Here's the drawing with two shaded views (mm, measured from the low corner). I have some questions. A direction names the side the tool comes from. Round coordinates to 2 decimals unless told otherwise and drop trailing zeros. Loops run counter-clockwise (first coordinate to the right, second up) from the corner with the lowest first, then second, coordinate; pieces in that order, holes last. Notation, with made-up numbers: (46.25, 24.25) -> (78.25, 24.25) arc R36 ccw to (78.25, 61.25) -> close; hole circle Ø3 at (20.5, 83). An arc over 180 degrees is marked (long way). Write item = value, one per line.
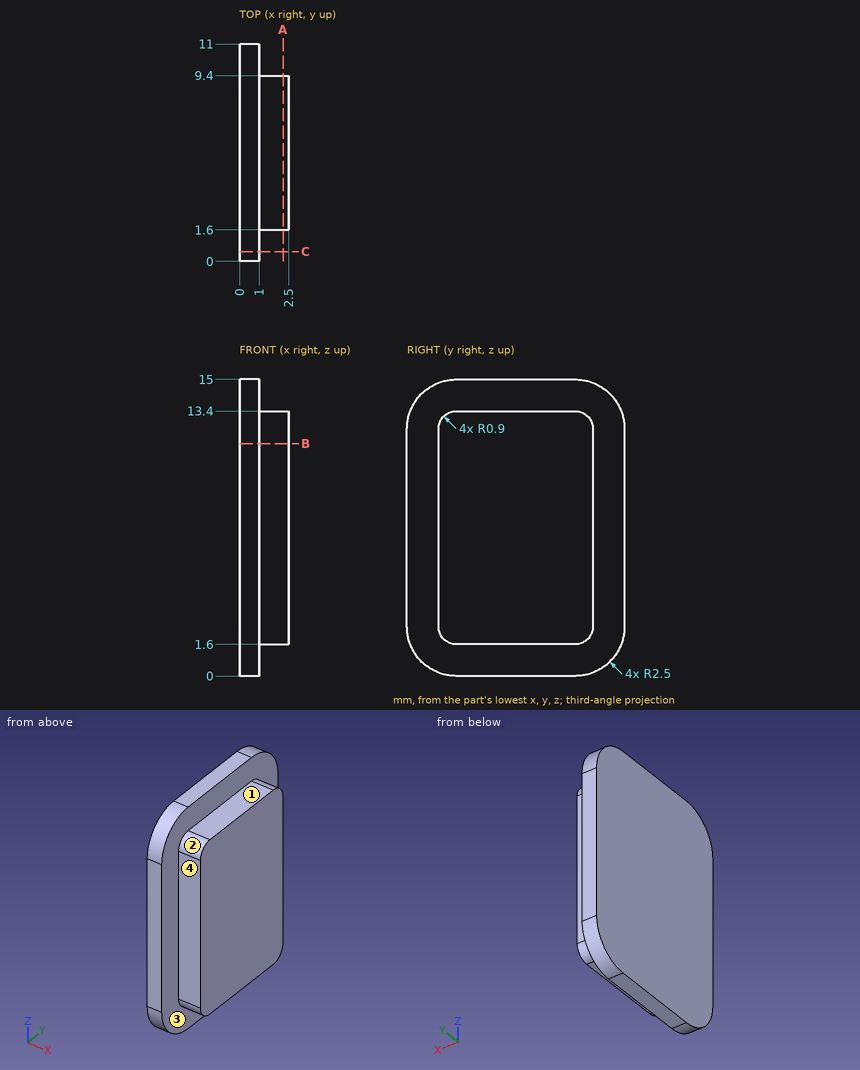
1. Suppose I cut it at C-C, the plane y = 0.5. List the corners of the cut face in (x, z) for me, and give its area (3 significant figures).
Entries:
outline = (0, 1) -> (1, 1) -> (1, 14) -> (0, 14) -> close
area = 13.0 mm²
2. Suppose I cut it at A-A, the plane x = 2.2. List the corners of the cut face in (y, z) for me, and give its area (3 significant figures).
Entries:
outline = (1.6, 2.5) arc R0.9 ccw to (2.5, 1.6) -> (8.5, 1.6) arc R0.9 ccw to (9.4, 2.5) -> (9.4, 12.5) arc R0.9 ccw to (8.5, 13.4) -> (2.5, 13.4) arc R0.9 ccw to (1.6, 12.5) -> close
area = 91.3 mm²
3. Suppose I cut it at B-B, the plane z = 11.75. List the corners of the cut face in (x, y) for me, and give its area (3 significant figures).
Entries:
outline = (0, 0) -> (1, 0) -> (1, 1.6) -> (2.5, 1.6) -> (2.5, 9.4) -> (1, 9.4) -> (1, 11) -> (0, 11) -> close
area = 22.7 mm²
4. I need wall thicknesses on line 1 (Y direction, x = 1.85, z = 6.75); line 2 (X direction, y = 1, z = 3.5); line 3 (Z direction, x = 2.15, y = 7.5). Which ranges of each line are inside material? Lowest first, please. Write a range as [from, to].
Entries:
line_1 = [1.6, 9.4]
line_2 = [0, 1]
line_3 = [1.6, 13.4]
5. For the marked faces 1, 2, 3 and 4, which set-ups out of +Z, -Z, +X, -X, +Y, -Y let a thin tool reach every point of the face, with its end or its side?
Entries:
face_1 = +Z, +X, +Y, -Y
face_2 = +Z, +X, -Y
face_3 = +X
face_4 = +Z, -Z, +X, -Y
6. I'm going to push flat-ended pins straight in: pin 1 (0.8 mm diameter, centred on x = 1.5, y = 5.5, fed in from -Z); pin 2 (2 mm diameter, centred on y = 5.5, z = 3.5, fed in from -X); pin 3 (0.8 mm diameter, centred on x = 1.5, z = 8, fed in from +Y). Where does each tip first touch, or does it pass through?
Entries:
pin_1 = 1.6
pin_2 = 0
pin_3 = 9.4
